from build123d import *

# Parameters (mm, degrees)
SKETCH_1_W      = 30
SKETCH_1_H      = 48
SKETCH_1_R      = 1
SKETCH_1_W_2    = 10
SKETCH_1_H_2    = 10
EXTRUDE_1_DEPTH = 1.6
FILLET_1_R      = 3
FILLET_2_R      = 1


with BuildPart() as part:
    # 草图1 → 凸台-拉伸1 (new body)
    with BuildSketch(Plane(origin=(0, 0, 0), x_dir=(1, 0, 0), z_dir=(0, 1, 0))):
        Rectangle(SKETCH_1_W, SKETCH_1_H)
        with Locations(Location((-12, -19, 0), (0, 0, 270))):
            Circle(SKETCH_1_R, mode=Mode.SUBTRACT)
        with Locations(Location((12, -19, 0), (0, 0, 270))):
            Circle(SKETCH_1_R, mode=Mode.SUBTRACT)
        with Locations((0, 9)):
            Rectangle(SKETCH_1_W_2, SKETCH_1_H_2, mode=Mode.SUBTRACT)
    extrude(amount=EXTRUDE_1_DEPTH)

    # 圆角1
    fillet_1_edges = [part.edges().sort_by_distance(p)[0] for p in [
        (15, 0.8, 24),
        (-15, 0.8, 24),
        (-15, 0.8, -24),
        (15, 0.8, -24),
    ]]
    fillet(fillet_1_edges, radius=FILLET_1_R)

    # 圆角2
    fillet_2_edges = [part.edges().sort_by_distance(p)[0] for p in [
        (5, 0.8, -4),
        (5, 0.8, -14),
        (-5, 0.8, -14),
        (-5, 0.8, -4),
    ]]
    fillet(fillet_2_edges, radius=FILLET_2_R)


solid = part.part
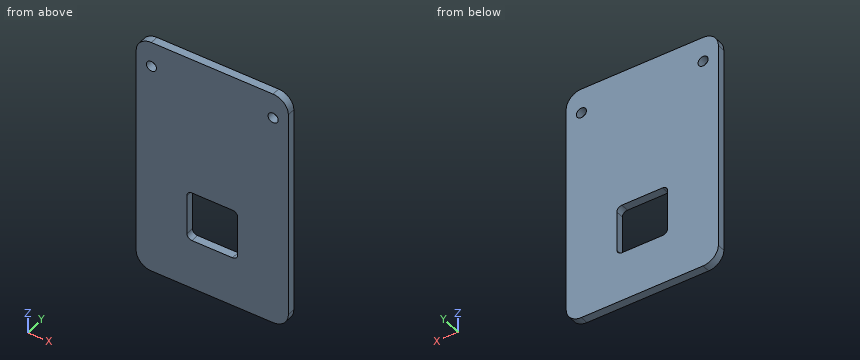
The model under review builds one solid part; all positions refer to its coordinate system, in mm. Round coordinates to 2 decimals unless told otherwise and drop trailing zeros. Loops run counter-clockwise (first coordinate to the right, second up) from the corner with the lowest first, then second, coordinate; pieces in that order, holes last. Notation, with made-up numbers: M -10,-0.75 L 43,-0.75 A27 cw 43,26.25 Z; hole C -31,-15 d6. An arc over 180 degrees is marked long. Answer as CSV lines item,"result".
1. We need section C-C (z = -12). Give the boundary of the cut face in (x, y).
Outcome:
outline,"M -15,0 L -5,0 L -5,1.6 L -15,1.6 Z; M 5,0 L 15,0 L 15,1.6 L 5,1.6 Z"
2. We need section B-B (z = 19). Give the boundary of the cut face in (x, y).
Outcome:
outline,"M -15,0 L -13,0 L -13,1.6 L -15,1.6 Z; M -11,0 L 11,0 L 11,1.6 L -11,1.6 Z; M 13,0 L 15,0 L 15,1.6 L 13,1.6 Z"
3. To check wall thickness, follow L1, parallel to X at y = 0.75, z = 19; L2, parallel to Z at x = -1.75, y = 0.95; L3, parallel to Z at x = 12.5, y = 0.5. State the ranges of each line that lie inside material, in increasing order. Write a range as [from, to].
Outcome:
L1,"x = [-15, -13], [-11, 11], [13, 15]"
L2,"z = [-24, -14], [-4, 24]"
L3,"z = [-23.96, 18.13], [19.87, 23.96]"
4. Insertion check: pin 1 Ø3 at (x, z) = (-12, 19) entering from +Y. The pin has a flat end and moves straight along its axis. Give the tip position at first contact, or say it passes through.
Outcome:
pin 1,"stops at y = 1.6"
5. We need section A-A (y = 0.35). Give the boundary of the cut face in (x, z), plus the area to 3 significant figures.
Outcome:
outline,"M -15,-21 A3 ccw -12,-24 L 12,-24 A3 ccw 15,-21 L 15,21 A3 ccw 12,24 L -12,24 A3 ccw -15,21 Z; hole C -12,19 d2; hole M -5,-13 A1 ccw -4,-14 L 4,-14 A1 ccw 5,-13 L 5,-5 A1 ccw 4,-4 L -4,-4 A1 ccw -5,-5 Z; hole C 12,19 d2"
area,"1,330 mm2"
